```python
from build123d import *

# Parameters (mm, degrees)
SKETCH1_W               = 19.05
SKETCH1_H               = 19.05
SKETCH1_W_2             = 15.875
SKETCH1_H_2             = 15.875
BOSS_EXTRUDE1_DEPTH     = 609.6
SKETCH3_R               = 3.175
CUT_EXTRUDE1_DEPTH      = 610.971956835
SKETCH4_R               = 3.175
CUT_EXTRUDE2_DEPTH      = 610.971956835
CUT_EXTRUDE4_DEPTH      = 610.971956835
CUT_EXTRUDE4_DEPTH_BACK = 610.971956835
SKETCH7_R               = 3.175


with BuildPart() as part:
    # Sketch1 → Boss-Extrude1 (new, symmetric)
    with BuildSketch(Plane.XY):
        Rectangle(SKETCH1_W, SKETCH1_H)
        Rectangle(SKETCH1_W_2, SKETCH1_H_2, mode=Mode.SUBTRACT)
    extrude(amount=BOSS_EXTRUDE1_DEPTH, both=True)

    # Sketch3 → Cut-Extrude1 (cut, through all)
    with BuildSketch(Plane(origin=(9.525, 0, 0), x_dir=(0, 0, -1), z_dir=(1, 0, 0))):
        with Locations((-571.5, 0)):
            Circle(SKETCH3_R)
        with Locations((-596.9, 0)):
            Circle(SKETCH3_R)
    extrude(amount=-CUT_EXTRUDE1_DEPTH, mode=Mode.SUBTRACT)

    # Sketch4 → Cut-Extrude2 (cut, through all)
    with BuildSketch(Plane.ZY.offset(9.525)):
        with Locations((444.5, 0)):
            Circle(SKETCH4_R)
        with Locations((419.1, 0)):
            Circle(SKETCH4_R)
    extrude(amount=-CUT_EXTRUDE2_DEPTH, mode=Mode.SUBTRACT)

    # Sketch7 → Cut-Extrude4 (cut, two sides: drawn at the far end of the back side and taken through both)
    with BuildSketch(Plane.XZ.offset(9.525).offset(-CUT_EXTRUDE4_DEPTH_BACK)):
        with Locations(Location((0, 292.1, 0), (0, 0, 90))):
            Circle(SKETCH7_R)
        with Locations(Location((0, 66.675, 0), (0, 0, 90))):
            Circle(SKETCH7_R)
    extrude(amount=CUT_EXTRUDE4_DEPTH + CUT_EXTRUDE4_DEPTH_BACK, mode=Mode.SUBTRACT)


solid = part.part
```
The listing builds one solid part. Answer for the finished solid, in the listing's coordinates (mm). Coordinates: 2 decimals unless noted, no trailing zeros. Loops run counter-clockwise (first coordinate to the right, second up) from the corner with the lowest first, then second, coordinate; pieces in that order, holes last. Notation, with made-up numbers: (16.25, 83) -> (48.25, 83) arc R28 ccw to (48.25, 108) -> close; hole circle Ø5 at (82, 41.25). An arc over 180 degrees is marked (long way). Return JSON: item names as keys, results as strings. Group by question number.
(1) Determine the mould class of faces 1 (the flat face through (-9, 0, -609.6)), 2 (the flat face through (-9, 0, 609.6)), 3 (the flat face through (-9.525, 0, 9)) for opening direction Z: released by +Z, released by -Z, zero draft, split by the parting line, or undercut.
(2) A cutting plane is placed at B-B on y = 0. Count the separate pieces of the cut face and the enclosed holes in it, and give its area (3 significant figures).
(3) Find the intervals of material crossed by probe 1 along Y at (x, z) = (2, -552) (1 decimal); probe 2 along Y at (x, z) = (-8.45, 444.5) (3 decimals), in increasing order. Write a range as from..to.
(4) A cutting plane is placed at A-A on z = 313. Write down the section's boundary in (x, y) (1 decimal), and give its area (3 significant figures).
(5) Given pin 1 Ø7.5 at (y, z) = (0, 444.5) entering from -X (3 decimals); pin 2 Ø5 at (x, z) = (0, 66.675) entering from -Y, each flat-ended and moving along its own axis, determine where each tip first touches the part or whether it passes through.
The answers:
{
 "1": {"face 1": "released by -Z", "face 2": "released by +Z", "face 3": "zero draft"},
 "2": {"separate pieces": "10", "enclosed holes": "0", "area": "3,790 mm^2"},
 "3": {"probe 1": "y = -9.5..-7.9, 7.9..9.5", "probe 2": "y = -9.525..-3.175, 3.175..9.525"},
 "4": {"outline": "(-9.5, -9.5) -> (9.5, -9.5) -> (9.5, 9.5) -> (-9.5, 9.5) -> close; hole (-7.9, -7.9) -> (7.9, -7.9) -> (7.9, 7.9) -> (-7.9, 7.9) -> close", "area": "111 mm^2"},
 "5": {"pin 1": "stops at x = -9.525", "pin 2": "passes through"}
}
